Can you work these out from the model? Positions are in its coordinate system, mm. A direction names the side the tool comes from. Round coordinates to 2 decimals unless told otherwise and drop trailing zeros. Loops run counter-clockwise (first coordinate to the right, second up) from the corner with the lowest first, then second, coordinate; pieces in that order, holes last. Notation, with made-up numbers: (62, 17) -> (117, 17) arc R19 cw to (117, 47) -> close; hole circle Ø8 at (-21.75, 84). An arc over 180 degrees is marked (long way). Use a Markdown table: item, result.
from build123d import *

# Parameters (mm, degrees)
CONVERGING_FILLET_R   = 3.175
BOLT_HOLES_D          = 6.35
BOLT_HOLES_DEPTH      = 12.7
BOLT_HOLES_TIP        = 1.907732465
PIN_HOLES_D           = 3.175
PIN_HOLES_DEPTH       = 100
PIN_HOLES_CBORE_D     = 6.35
PIN_HOLES_CBORE_DEPTH = 6.35


with BuildPart() as part:
    # Sketch1 → Main Revolve (revolve)
    with BuildSketch(Plane.XY):
        with BuildLine():
            Line((-9.517884855, 29.85426414), (-9.517884855, 31.004317662))
            ThreePointArc((-9.517884855, 31.004317662), (-10.387063469, 33.747209355), (-12.677340956, 35.488919819))
            add(Edge.make_bspline(
                [(-41.275, 127), (-41.268873036, 126.161357833), (-41.222997706, 124.484568363), (-41.073369126, 121.078528782), (-40.722786085, 115.949040077), (-40.170467422, 109.939618965), (-39.360849464, 103.059106185), (-38.382227863, 96.200616774), (-37.230570221, 89.368983139), (-35.895631241, 82.570619969), (-34.35912374, 75.814773558), (-32.593807355, 69.114550244), (-30.558516971, 62.490757957), (-28.191269221, 55.976383127), (-25.683140783, 50.29180013), (-23.125834222, 45.592543641), (-20.711209845, 42.055498174), (-18.720317843, 39.685916503), (-17.052831983, 38.103539579), (-15.746862259, 37.100217478), (-14.77072941, 36.476537732), (-14.077416444, 36.090491664), (-13.464775463, 35.797858298), (-13.037564762, 35.6215562), (-12.773284859, 35.523215456), (-12.677340956, 35.488919819)],
                knots=[0, 0, 0, 0, 0, 0.030811657, 0.061623313, 0.125250249, 0.188877076, 0.252503727, 0.31613061, 0.379757458, 0.443384315, 0.507011165, 0.570638032, 0.634264894, 0.697891611, 0.761518516, 0.798698062, 0.830511144, 0.855003573, 0.875012249, 0.882965592, 0.890918935, 0.897534321, 0.904149707, 0.907892787, 0.907892787, 0.907892787, 0.907892787, 0.907892787], degree=4))
            Line((-41.275, 127), (-44.449999999, 127))
            add(Edge.make_bspline(
                [(-44.449999999, 127), (-44.444048095, 126.089867786), (-44.399723494, 124.270031311), (-44.256170835, 120.604636062), (-43.921206973, 115.098603125), (-43.395046361, 108.666141993), (-42.624644612, 101.314791698), (-41.691159468, 93.9823601), (-40.588904101, 86.673339257), (-39.305520483, 79.393738689), (-37.819617038, 72.152599105), (-36.098890328, 64.963007024), (-34.092981802, 57.847082032), (-31.766198141, 50.972017381), (-29.315037347, 45.128649076), (-26.838138987, 40.469327818), (-24.570330265, 37.178251455), (-22.783120415, 35.132973657), (-21.307300799, 33.836487802), (-20.194653885, 33.074782772), (-19.515295281, 32.700466394), (-19.20577242, 32.548791321), (-19.05, 32.47725184)],
                knots=[0, 0, 0, 0, 0, 0.033160808, 0.066321616, 0.133644696, 0.20096779, 0.268290787, 0.335613842, 0.40293693, 0.470260007, 0.537583094, 0.604906139, 0.672229114, 0.739552316, 0.801869766, 0.835531618, 0.86410438, 0.88489762, 0.900577549, 0.906888404, 0.913134212, 0.913134212, 0.913134212, 0.913134212, 0.913134212], degree=4))
            Line((-19.05, 32.47725184), (-19.049999999, 28.042086726))
            add(Edge.make_bspline(
                [(-40.132930327, 12.7), (-40.045800084, 12.849795641), (-39.61063411, 13.587366211), (-38.787730692, 14.889107917), (-37.49639122, 16.700465362), (-35.743276325, 18.799808382), (-33.828362814, 20.752874932), (-31.755293022, 22.538171222), (-29.765599353, 23.963838921), (-27.959230186, 25.046029913), (-26.389400219, 25.845449005), (-25.088892975, 26.420387951), (-23.81412329, 26.906738928), (-22.507881474, 27.32323595), (-21.192562324, 27.667064424), (-20.14685077, 27.874680732), (-19.448803378, 27.987030694), (-19.080597755, 28.037915662), (-19.049999999, 28.042086726)],
                knots=[0.281378447, 0.281378447, 0.281378447, 0.281378447, 0.281378447, 0.29580073, 0.352648866, 0.409496837, 0.466344885, 0.523192931, 0.580040954, 0.636888987, 0.669796212, 0.698220237, 0.726644255, 0.755068258, 0.783492282, 0.811916293, 0.840340301, 0.842913615, 0.842913615, 0.842913615, 0.842913615, 0.842913615], degree=4))
            Line((-40.132930327, 12.7), (-66.675, 12.7))
            Line((-66.675, 12.7), (-66.675, 0))
            Line((-66.675, 0), (-41.275, 0))
            add(Edge.make_bspline(
                [(-41.275, 0), (-41.27404827, 0.048633732), (-41.270265816, 0.145822286), (-41.249886429, 0.420698051), (-41.184454538, 0.952068232), (-41.045697232, 1.718226005), (-40.803050388, 2.710615824), (-40.471359514, 3.795919992), (-40.073863441, 4.892829094), (-39.58250679, 6.074812663), (-38.909330489, 7.49520986), (-38.013176032, 9.129802593), (-36.850990459, 10.946036297), (-35.454742127, 12.816921248), (-33.931439219, 14.585782904), (-32.290383905, 16.245919147), (-30.54007116, 17.790421623), (-28.688732636, 19.212251207), (-26.744575764, 20.504343604), (-24.716209135, 21.659734331), (-22.61250234, 22.671709773), (-20.443220111, 23.533972634), (-18.496293348, 24.152467466), (-16.799886455, 24.58239915), (-15.513443264, 24.843608525), (-14.65819574, 24.990901269), (-14.086451577, 25.07519752), (-13.804404299, 25.113562074), (-13.666257288, 25.131526207)],
                knots=[0, 0, 0, 0, 0, 0.004014849, 0.008029698, 0.022747096, 0.044177712, 0.068247366, 0.092316927, 0.116386463, 0.140456137, 0.173883837, 0.222022894, 0.270162138, 0.318301135, 0.366440287, 0.41457937, 0.462718533, 0.510857613, 0.558996755, 0.607135854, 0.655274938, 0.703414059, 0.751553162, 0.775622711, 0.799692261, 0.811727037, 0.823244082, 0.823244082, 0.823244082, 0.823244082, 0.823244082], degree=4))
            ThreePointArc((-13.666257288, 25.131526207), (-10.702243662, 26.711285957), (-9.517884855, 29.85426414))
        make_face()
    revolve(axis=Axis((0, 0, 0), (0, 1, 0)))

    # Converging Fillet
    converging_fillet_edges = [part.edges().sort_by_distance(p)[0] for p in [
        (40.132930327, 12.7, 0),
    ]]
    fillet(converging_fillet_edges, radius=CONVERGING_FILLET_R)

    # Bolt Holes
    with Locations(Plane(origin=(0, 12.7, 0), x_dir=(1, 0, 0), z_dir=(0, 1, 0))):
        with Locations((-58.42, 0), (-41.309178157, 41.309178157), (0, 58.42), (41.309178157, 41.309178157), (58.42, 0), (41.309178157, -41.309178157), (0, -58.42), (-41.309178157, -41.309178157)):
            Hole(BOLT_HOLES_D / 2, depth=BOLT_HOLES_DEPTH)
            with Locations((0, 0, -(BOLT_HOLES_DEPTH + BOLT_HOLES_TIP / 2))):  # 118° drill point
                Cone(0, BOLT_HOLES_D / 2, BOLT_HOLES_TIP, mode=Mode.SUBTRACT)

    # Pin Holes
    with Locations(Plane(origin=(0, 0, 0), x_dir=(-1, 0, 0), z_dir=(0, -1, 0))):
        with Locations((-22.356366119, 53.973042289), (22.356366119, -53.973042289)):
            CounterBoreHole(PIN_HOLES_D / 2, PIN_HOLES_CBORE_D / 2, PIN_HOLES_CBORE_DEPTH, depth=PIN_HOLES_DEPTH)


solid = part.part
1. I need wall thicknesses on line 1 (Y direction, x = -17, z = 48); line 2 (Z direction, x = 0, y = 5) (3 decimals); line 3 (Z direction, x = 16, y = 6). Which ranges of each line are inside material? Lowest first, please.
Answer sheet:
| item | result |
|---|---|
| line 1 | y = 0 to 12.7 |
| line 2 | z = -66.675 to -61.595, -55.245 to -40.02, 40.02 to 55.245, 61.595 to 66.675 |
| line 3 | z = -64.73 to -36.23, 36.23 to 64.73 |
2. I want a section at B-B (x = 0). State how many separate pieces and enclosed holes the cut face has, plus the area to 3 significant figures.
Answer sheet:
| item | result |
|---|---|
| separate pieces | 4 |
| enclosed holes | 0 |
| area | 1,770 mm² |
3. Will these pins go through, and if not, where does the flat tip stop? pin 1 Ø8.5 at (x, z) = (-58.42, 0) entering from -Y; pin 2 Ø4 at (x, z) = (22.36, -53.97) entering from +Y; pin 3 Ø3 at (x, y) = (-10, 69.5) entering from -Z; pin 4 Ø1.9 at (x, z) = (-24, 53.5) entering from -Y.
Answer sheet:
| item | result |
|---|---|
| pin 1 | stops at y = 0 |
| pin 2 | stops at y = 12.7 |
| pin 3 | stops at z = -36.32 |
| pin 4 | stops at y = 6.35 |
4. If we mould it in two halves opening along X, with no side actions, what happens to faces 1 (the flat face through (-31, 12.7, -29)), 2 (the cylindrical face through (15.12, 30.23, -11.59)), 3 (the cylindrical face through (-61.45, 6.26, -0.95))? For each: +X half, -X half, draft (parallel to the pull), parting line (faces both ways), or undercut.
Answer sheet:
| item | result |
|---|---|
| face 1 | draft |
| face 2 | parting line |
| face 3 | undercut |
5. Which directions (+Z, -Z, +X, -X, +Y, -Y) give clear straight access to the entire face, cutting with the end or side of a thin tool? Please do faces 4 (the cylindrical face through (-63.596, 6.261, 20.027)), 5 (the cylindrical face through (-24.063, 3.131, 51.296)).
Answer sheet:
| item | result |
|---|---|
| face 4 | +Y, -Y |
| face 5 | -Y |
6. I want a section at A-A (x = -58.42). Please give me the cut outline in (y, z) (3 decimals), plus the area to 3 significant figures.
Answer sheet:
| item | result |
|---|---|
| outline | (0, -32.135) -> (12.7, -32.135) -> (12.7, -3.175) -> (0, -3.175) -> close; (0, 3.175) -> (12.7, 3.175) -> (12.7, 32.135) -> (0, 32.135) -> close |
| area | 736 mm² |
